For this review, take the finished solid that the model builds, in its own axes (mm). Face numbers are marked on the shaded views. A direction names the side the tool comes from. Give positions to 0.01 mm unless a question says otherwise; leave off trailing zeros. Write each loop counter-clockwise with the first axis right and the second up, starting at its lowest first coordinate (ties: lowest second). Pieces come first, ordered by that corner, then holes. Notation, with made-up numbers: M 67,17 L 71,17 A27 ccw 71,39 Z; hole C 49,22.5 d11. An arc over 180 degrees is marked long. One line per item, written item: value. Start each with the question number.
Item 1: Consider section A-A, the plane x = 22.5. Write out the cut boundary in (y, z).
Item 2: Tool access review of the marked faces 4, 5 and 6: name each direction out of +Z, -Z, +X, -X, +Y, -Y from which nothing blocks a thin tool from reaching the whole face with its end or side.
Item 3: Mouldability with a two-part tool opening along Y and no side actions: class the marked faces 1, 2 and 3 as released by +Y, released by -Y, zero draft, split by the parting line, or undercut.
Item 4: Consider section C-C, the plane z = 12. Write out the cut boundary in (x, y), and give its area (3 significant figures).
Item 5: Consider section B-B, the plane y = 15.5. Write out the cut boundary in (x, z), and give its area (3 significant figures).
Item 6: To check wall thickness, follow probe 1 along X at (y, z) = (0.5, 6); probe 2 along X at (y, z) = (-0.5, 2.75); probe 3 along X at (y, z) = (-2, 0.5). State the ranges of each line that lie inside material, in increasing order.
Item 7: Consider section D-D, the plane x = 0. Write out the cut boundary in (y, z).
Item 8: Clearance check with flat-ended pins moving along their axes: pin 1 Ø7.5 at (x, y) = (48.5, -7.5) entering from -Z; pin 2 Ø6 at (x, z) = (6, 0.5) entering from +Y; pin 3 Ø3 at (x, z) = (43, 7.5) entering from +Y. State where each tip first meets the part, or that it passes through.
```python
from build123d import *

# Parameters (mm, degrees)
BOSS_EXTRUDE1_DEPTH          = 15
SKETCH6_R                    = 3.5
SKETCH6_R_2                  = 1.8288
HUB_MOUNT_HOLE_PATTERN_DEPTH = 62.660360038
SKETCH7_R                    = 1.75
SKETCH7_R_2                  = 3.25
MOTOR_HOLE_PATTERN_DEPTH     = 62.660360038
SKETCH8_R                    = 18.75
MOTOR_CUTOUT_DEPTH           = 5
HUB_START                    = -7
HUB_MOUNT_CUTOUT_DEPTH       = 7
SKETCH10_R                   = 5
BOSS_EXTRUDE2_DEPTH          = 5.5
LINKAGE_PIN_HOLE_DEPTH       = 62.660360038
LINKAGE_PIN_HOLE_DEPTH_BACK  = 62.660360038
SKETCH12_R                   = 1.55
CHAMFER1_SIZE                = 2.75
SKETCH13_R                   = 6.1
CUT_EXTRUDE7_DEPTH           = 7.1
SKETCH14_R                   = 7
CUT_EXTRUDE8_DEPTH           = 3
SKETCH15_R                   = 3.5
CUT_EXTRUDE9_DEPTH           = 5
CUT_EXTRUDE10_DEPTH          = 62.312722986
CUT_EXTRUDE10_DEPTH_BACK     = 3
SKETCH16_R                   = 3
CUT_EXTRUDE12_DEPTH          = 7
BOSS_EXTRUDE3_REACH          = 63.784
CUT_EXTRUDE13_DEPTH          = 62.660360038
CUT_EXTRUDE13_DEPTH_BACK     = 3
SKETCH19_R                   = 4
FILLET1_R                    = 5


with BuildPart() as part:
    # Sketch2 → Boss-Extrude1 (new body)
    with BuildSketch(Plane.XY):
        with BuildLine():
            Line((-2.971428571, 12.655852885), (30.2, 20.444070045))
            ThreePointArc((30.2, 20.444070045), (56, 0), (30.2, -20.444070045))
            Line((30.2, -20.444070045), (-2.971428571, -12.655852885))
            ThreePointArc((-2.971428571, -12.655852885), (-13, 0), (-2.971428571, 12.655852885))
        make_face()
    extrude(amount=BOSS_EXTRUDE1_DEPTH)

    # Sketch6 → hub mount hole pattern (cut, through all)
    with BuildSketch(Plane.XY.offset(15)):
        Circle(SKETCH6_R)
        with Locations((-6.914797213, 6.914797213)):
            Circle(SKETCH6_R_2)
        with Locations((6.914797213, 6.914797213)):
            Circle(SKETCH6_R_2)
        with Locations((6.914797213, -6.914797213)):
            Circle(SKETCH6_R_2)
        with Locations((-6.914797213, -6.914797213)):
            Circle(SKETCH6_R_2)
    extrude(amount=-HUB_MOUNT_HOLE_PATTERN_DEPTH, mode=Mode.SUBTRACT)

    # Sketch7 → motor hole pattern (cut, through all)
    with BuildSketch(Plane.XY.offset(15)):
        with Locations((21.576606241, 7.75)):
            Circle(SKETCH7_R)
        with Locations((35, 15.5)):
            Circle(SKETCH7_R)
        with Locations((48.423393759, 7.75)):
            Circle(SKETCH7_R)
        with Locations((48.423393759, -7.75)):
            Circle(SKETCH7_R)
        with Locations((35, -15.5)):
            Circle(SKETCH7_R)
        with Locations((21.576606241, -7.75)):
            Circle(SKETCH7_R)
        with Locations((42, 0)):
            Circle(SKETCH7_R_2)
    extrude(amount=-MOTOR_HOLE_PATTERN_DEPTH, mode=Mode.SUBTRACT)

    # Sketch8 → motor cutout (cut)
    with BuildSketch(Plane.XY.offset(15)):
        with Locations((35, 0)):
            Circle(SKETCH8_R)
    extrude(amount=-MOTOR_CUTOUT_DEPTH, mode=Mode.SUBTRACT)

    # Sketch9 → hub mount cutout (cut)
    with BuildSketch(Plane.XY.offset(15).offset(HUB_START)):
        with BuildLine():
            ThreePointArc((-7.281143007, 10.769631215), (-13, 0), (-7.281143007, -10.769631215))
            ThreePointArc((-7.281143007, -10.769631215), (-6.15529138, -10.711783559), (-5.093815501, -10.332103173))
            ThreePointArc((-5.093815501, -10.332103173), (-4.17580433, -10.057753531), (-3.223255475, -10.161014917))
            ThreePointArc((-3.223255475, -10.161014917), (0, -10.66), (3.223255475, -10.161014917))
            ThreePointArc((3.223255475, -10.161014917), (4.17580433, -10.057753531), (5.093815501, -10.332103173))
            ThreePointArc((5.093815501, -10.332103173), (9.652858062, -9.652858062), (10.332103173, -5.093815501))
            ThreePointArc((10.332103173, -5.093815501), (10.057753531, -4.17580433), (10.161014917, -3.223255475))
            ThreePointArc((10.161014917, -3.223255475), (10.66, 0), (10.161014917, 3.223255475))
            ThreePointArc((10.161014917, 3.223255475), (10.057753531, 4.17580433), (10.332103173, 5.093815501))
            ThreePointArc((10.332103173, 5.093815501), (9.652858062, 9.652858062), (5.093815501, 10.332103173))
            ThreePointArc((5.093815501, 10.332103173), (4.17580433, 10.057753531), (3.223255475, 10.161014917))
            ThreePointArc((3.223255475, 10.161014917), (0, 10.66), (-3.223255475, 10.161014917))
            ThreePointArc((-3.223255475, 10.161014917), (-4.17580433, 10.057753531), (-5.093815501, 10.332103173))
            ThreePointArc((-5.093815501, 10.332103173), (-6.15529138, 10.711783559), (-7.281143007, 10.769631215))
        make_face()
    extrude(amount=HUB_MOUNT_CUTOUT_DEPTH, mode=Mode.SUBTRACT)

    # Sketch10 → Boss-Extrude2 (add)
    with BuildSketch(Plane(origin=(0, 0, 0), x_dir=(-1, 0, 0), z_dir=(0, 0, -1))):
        with Locations(Location((-11, 0, 0), (0, 0, 180))):
            Circle(SKETCH10_R)
    extrude(amount=BOSS_EXTRUDE2_DEPTH)

    # Sketch12 → Linkage pin hole (cut, two sides: drawn at the far end of the back side and taken through both)
    with BuildSketch(Plane.XY.offset(-LINKAGE_PIN_HOLE_DEPTH_BACK)):
        with Locations((11, 0)):
            Circle(SKETCH12_R)
    extrude(amount=LINKAGE_PIN_HOLE_DEPTH + LINKAGE_PIN_HOLE_DEPTH_BACK, mode=Mode.SUBTRACT)

    # Chamfer1
    chamfer1_edges = [part.edges().sort_by_distance(p)[0] for p in [
        (6, 0, -5.5),
    ]]
    chamfer(chamfer1_edges, length=CHAMFER1_SIZE)

    # Sketch13 → Cut-Extrude7 (cut)
    with BuildSketch(Plane.XY.offset(10)):
        with Locations((42, 0)):
            Circle(SKETCH13_R)
    extrude(amount=-CUT_EXTRUDE7_DEPTH, mode=Mode.SUBTRACT)

    # Sketch14 → Cut-Extrude8 (cut)
    with BuildSketch(Plane.XY.offset(8)):
        Circle(SKETCH14_R)
    extrude(amount=-CUT_EXTRUDE8_DEPTH, mode=Mode.SUBTRACT)

    # Sketch15 → Cut-Extrude9 (cut)
    with BuildSketch(Plane(origin=(0, 0, 0), x_dir=(-1, 0, 0), z_dir=(0, 0, -1))):
        with Locations((-21.576606241, -7.75)):
            Circle(SKETCH15_R)
        with Locations((-35, -15.5)):
            Circle(SKETCH15_R)
        with Locations((-48.423393759, -7.75)):
            Circle(SKETCH15_R)
        with Locations((-48.423393759, 7.75)):
            Circle(SKETCH15_R)
        with Locations((-35, 15.5)):
            Circle(SKETCH15_R)
        with Locations((-21.576606241, 7.75)):
            Circle(SKETCH15_R)
    extrude(amount=-CUT_EXTRUDE9_DEPTH, mode=Mode.SUBTRACT)

    # Sketch16 → Cut-Extrude10 (cut, two sides: drawn at the far end of the back side and taken through both)
    with BuildSketch(Plane.XY.offset(8).offset(-CUT_EXTRUDE10_DEPTH_BACK)):
        with Locations(Location((11, 0, 0), (0, 0, 104.35596801))):
            Circle(SKETCH16_R)
    extrude(amount=CUT_EXTRUDE10_DEPTH + CUT_EXTRUDE10_DEPTH_BACK, mode=Mode.SUBTRACT)

    # Sketch17 → Cut-Extrude12 (cut)
    with BuildSketch(Plane.XY.offset(10)):
        with BuildLine():
            ThreePointArc((39.857142857, 8.741176309), (25, 0), (39.857142857, -8.741176309))
            ThreePointArc((39.857142857, -8.741176309), (33, 0), (39.857142857, 8.741176309))
        make_face()
    extrude(amount=-CUT_EXTRUDE12_DEPTH, mode=Mode.SUBTRACT)

    # Sketch18 → Boss-Extrude3 (add, up to next)
    with BuildSketch(Plane.XY.offset(10), mode=Mode.PRIVATE) as boss_extrude3_sk1:
        with BuildLine():
            Line((27.471985333, -6.582476371), (33.992343948, -4.108216712))
            ThreePointArc((33.992343948, -4.108216712), (33.585458911, -3.193039032), (33.282779719, -2.238318693))
            Line((33.282779719, -2.238318693), (26.280269544, -4.895538864))
            ThreePointArc((26.280269544, -4.895538864), (26.83245784, -5.769857456), (27.471985333, -6.582476371))
        make_face()
    boss_extrude3_tool1 = extrude(boss_extrude3_sk1.sketch, amount=-BOSS_EXTRUDE3_REACH, mode=Mode.PRIVATE) - part.part
    # Sketch18 → Boss-Extrude3 (add, up to next)
    with BuildSketch(Plane.XY.offset(10), mode=Mode.PRIVATE) as boss_extrude3_sk2:
        with BuildLine():
            Line((27.471985333, 6.582476371), (33.992343948, 4.108216712))
            ThreePointArc((33.992343948, 4.108216712), (33.585458911, 3.193039032), (33.282779719, 2.238318693))
            Line((33.282779719, 2.238318693), (26.280269544, 4.895538864))
            ThreePointArc((26.280269544, 4.895538864), (26.83245784, 5.769857456), (27.471985333, 6.582476371))
        make_face()
    boss_extrude3_tool2 = extrude(boss_extrude3_sk2.sketch, amount=-BOSS_EXTRUDE3_REACH, mode=Mode.PRIVATE) - part.part
    add(boss_extrude3_tool1.solids().sort_by_distance((30.216616, -4.45872, 10))[0])
    add(boss_extrude3_tool2.solids().sort_by_distance((30.216616, 4.45872, 10))[0])

    # Sketch19 → Cut-Extrude13 (cut, two sides: drawn at the far end of the back side and taken through both)
    with BuildSketch(Plane(origin=(0, 0, 0), x_dir=(-1, 0, 0), z_dir=(0, 0, -1)).offset(-CUT_EXTRUDE13_DEPTH_BACK)):
        with Locations(Location((-6.914797213, -6.914797213, 0), (0, 0, 90.325769881))):
            Circle(SKETCH19_R)
        with Locations(Location((-6.914797213, 6.914797213, 0), (0, 0, 269.674230119))):
            Circle(SKETCH19_R)
        with Locations((6.914797213, 6.914797213)):
            Circle(SKETCH19_R)
        with Locations((6.914797213, -6.914797213)):
            Circle(SKETCH19_R)
    extrude(amount=CUT_EXTRUDE13_DEPTH + CUT_EXTRUDE13_DEPTH_BACK, mode=Mode.SUBTRACT)

    # Fillet1
    # the kernel refuses this fillet: 5 mm, written as the material it adds along each edge
    with BuildSketch(Plane(origin=(11, 0, 0), x_dir=(-0.9999950652018581, 0.003141587485879405, 0), z_dir=(-0.003141587485879405, -0.9999950652018581, 0))) as fillet1_piece_1_section:
        with BuildLine():
            CenterArc((9.465142775, 5), FILLET1_R, 206.74368395, 63.25631605)
            Line((9.465142775, 0), (9.465142775, -0.1))
            Line((9.465142775, -0.1), (5, -0.1))
            Line((5, -0.1), (4.9, 0))
            ThreePointArc((4.9, 0), (4.9, 1.375), (4.910697145, 2.705))
            Line((4.910697145, 2.705), (5, 2.75))
        make_face()
    fillet1_piece_1 = revolve(axis=Axis((11, 0, 0), (0, 0, -1)), revolution_arc=359.64, mode=Mode.PRIVATE)
    fillet1_piece_1 = fillet1_piece_1 - Plane(origin=(6.914797213, -6.914797213, -0.76540866), x_dir=(0.0056857263926290095, 0.9999838361270588, 0), z_dir=(0, 0, 1)) * Cylinder(4, 38, mode=Mode.PRIVATE)
    fillet1_piece_1 = fillet1_piece_1 - Plane(origin=(6.914797213, 6.914797213, -0.76540866), x_dir=(0.00568572639262881, -0.9999838361270588, 0), z_dir=(0, 0, 1)) * Cylinder(4, 38, mode=Mode.PRIVATE)
    fillet1_piece_1 = fillet1_piece_1 - Plane(origin=(0, 0, -0.76540866), x_dir=(1, 0, 0), z_dir=(0, 0, 1)) * Cylinder(3.5, 38, mode=Mode.PRIVATE)
    add(fillet1_piece_1)
    with BuildSketch(Plane(origin=(11, 0, 0), x_dir=(0.9593586032510993, -0.2821897772211103, 0), z_dir=(0.2821897772211103, 0.9593586032510993, 0))) as fillet1_piece_2_section:
        with BuildLine():
            CenterArc((9.465142775, 5), FILLET1_R, 206.74368395, 63.25631605)
            Line((9.465142775, 0), (9.465142775, -0.1))
            Line((9.465142775, -0.1), (5, -0.1))
            Line((5, -0.1), (4.9, 0))
            ThreePointArc((4.9, 0), (4.9, 1.375), (4.910697145, 2.705))
            Line((4.910697145, 2.705), (5, 2.75))
        make_face()
    fillet1_piece_2 = revolve(axis=Axis((11, 0, 0), (0, 0, -1)), revolution_arc=327.218117947, mode=Mode.PRIVATE)
    fillet1_piece_2 = fillet1_piece_2 - Plane(origin=(6.914797213, -6.914797213, -0.749324739), x_dir=(0.0056857263926290095, 0.9999838361270588, 0), z_dir=(0, 0, 1)) * Cylinder(4, 38, mode=Mode.PRIVATE)
    fillet1_piece_2 = fillet1_piece_2 - Plane(origin=(6.914797213, 6.914797213, -0.749324739), x_dir=(0.00568572639262881, -0.9999838361270588, 0), z_dir=(0, 0, 1)) * Cylinder(4, 38, mode=Mode.PRIVATE)
    fillet1_piece_2 = fillet1_piece_2 - Plane(origin=(0, 0, -0.749324739), x_dir=(1, 0, 0), z_dir=(0, 0, 1)) * Cylinder(3.5, 38, mode=Mode.PRIVATE)
    add(fillet1_piece_2)


solid = part.part
```
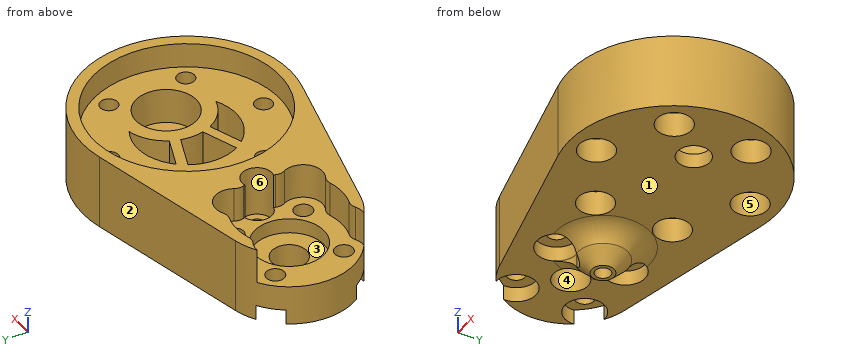
Model answer:
1. outline: M -18.64,0 L -11.13,0 L -11.13,5 L -9.24,5 L -9.24,10 L -13.98,10 L -13.98,15 L -18.64,15 Z; M -6.26,5 L -4.37,5 L -4.37,0 L 4.37,0 L 4.37,5 L 6.26,5 L 6.26,10 L -6.26,10 Z; M 9.24,5 L 11.13,5 L 11.13,0 L 18.64,0 L 18.64,15 L 13.98,15 L 13.98,10 L 9.24,10 Z
2. face 4: +Z, -Z
2. face 5: -Z
2. face 6: +Z
3. face 1: zero draft
3. face 2: released by +Y
3. face 3: undercut
4. outline: M -7.28,-10.77 A13 ccw -2.97,-12.66 L 30.2,-20.44 A21 ccw long 30.2,20.44 L -2.97,12.66 A13 ccw -7.28,10.77 A3.87 cw -5.09,10.33 A2.42 ccw -3.22,10.16 A10.66 cw 3.22,10.16 A2.42 ccw 5.09,10.33 A3.87 cw 10.33,5.09 A2.42 ccw 10.16,3.22 A10.66 cw 10.26,2.91 A3 cw long 10.26,-2.91 A10.66 cw 10.16,-3.22 A2.42 ccw 10.33,-5.09 A3.87 cw 5.09,-10.33 A2.42 ccw 3.22,-10.16 A10.66 cw -3.22,-10.16 A2.42 ccw -5.09,-10.33 A3.87 cw Z; hole C 35,0 d37.5
4. area: 603 mm2
5. outline: M 9.14,0 L 31.5,0 L 31.5,5 L 33.25,5 L 33.25,10 L 24.45,10 L 24.45,15 L 9.14,15 Z; M 36.75,5 L 38.5,5 L 38.5,0 L 49.17,0 L 49.17,15 L 45.55,15 L 45.55,10 L 36.75,10 Z
5. area: 442 mm2
6. probe 1: x = -12.99 to -6.98, 6.98 to 8.04, 13.96 to 25.01, 33.01 to 35.92, 48.08 to 55.99
6. probe 2: x = -12.99 to -3.46, 3.46 to 9.53, 12.47 to 38.79, 45.21 to 55.99
6. probe 3: x = -12.85 to -2.87, 2.87 to 39.44, 44.56 to 55.9
7. outline: M -13.35,0 L -3.5,0 L -3.5,5 L -7,5 L -7,8 L -10.66,8 L -10.66,15 L -13.35,15 Z; M 3.5,0 L 13.35,0 L 13.35,15 L 10.66,15 L 10.66,8 L 7,8 L 7,5 L 3.5,5 Z
8. pin 1: stops at z = 0
8. pin 2: stops at y = 15.47
8. pin 3: stops at y = 19.97
